from build123d import *

# Parameters (mm, degrees)
SKETCH1_R           = 4.8
SKETCH1_R_2         = 1.5
SKETCH1_R_3         = 4.5
BOSS_EXTRUDE1_DEPTH = 4


with BuildPart() as part:
    # Sketch1 → Boss-Extrude1 (new body)
    # profile 1 of 5: a face of its own
    with BuildSketch(Plane.XY):
        Polygon((-125, 88.228571429), (-125, 63.142246191), (94.856226429, -83.428571429), (123.942857143, -83.428571429), (123.942857143, 88.228571429), align=None)
        with Locations((107.142857143, -71.428571429)):
            Circle(SKETCH1_R, mode=Mode.SUBTRACT)
        with Locations((-107.142857143, 71.428571429)):
            Circle(SKETCH1_R, mode=Mode.SUBTRACT)
        with Locations((21.832408692, 6.152026506)):
            Circle(SKETCH1_R_2, mode=Mode.SUBTRACT)
        with Locations((37.332408692, 21.652026506)):
            Circle(SKETCH1_R_3, mode=Mode.SUBTRACT)
        with Locations((52.832408692, 6.152026506)):
            Circle(SKETCH1_R_2, mode=Mode.SUBTRACT)
        with Locations((21.832408692, 37.152026506)):
            Circle(SKETCH1_R_2, mode=Mode.SUBTRACT)
        with Locations((52.832408692, 37.152026506)):
            Circle(SKETCH1_R_2, mode=Mode.SUBTRACT)
        with Locations((107.142857143, 71.428571429)):
            Circle(SKETCH1_R, mode=Mode.SUBTRACT)
    # profile 2 of 5: a face of its own
    with BuildSketch(Plane.XY):
        with Locations((21.832408692, 6.152026506)):
            Circle(SKETCH1_R_2)
    # profile 3 of 5: a face of its own
    with BuildSketch(Plane.XY):
        with Locations((21.832408692, 37.152026506)):
            Circle(SKETCH1_R_2)
    # profile 4 of 5: a face of its own
    with BuildSketch(Plane.XY):
        with Locations((52.832408692, 37.152026506)):
            Circle(SKETCH1_R_2)
    # profile 5 of 5: a face of its own
    with BuildSketch(Plane.XY):
        with Locations((52.832408692, 6.152026506)):
            Circle(SKETCH1_R_2)
    extrude(amount=BOSS_EXTRUDE1_DEPTH)


solid = part.part
Could you check a few things on this model? Use its own coordinates, in mm. Give positions to 0.01 mm unless a question says otherwise; leave off trailing zeros. Order: outer loops, then holes, each group sorted by start corner. A loop starts at its lowest first (then second) coordinate and runs counter-clockwise, first axis right, second up.
Item 1: I need wall thicknesses on line 1 (Y direction, x = 110.5, z = 0.9); line 2 (X direction, y = 48, z = 3.25); line 3 (X direction, y = 63, z = 3.85). Which ranges of each line are inside material? Lowest first, please.
Item 2: If we section it at A-A, the plane z = 1.6: Write out the boundary of the cut face in (x, y), plus the area to 3 significant figures.
Item 3: If we section it at B-B, the plane y = 31: Write out the boundary of the cut face in (x, z).
Item 4: I'm going to push a flat-ended pin straight in: pin 1 (1 mm diameter, centred on x = 81.5, z = 3.5, fed in from -Y). Where does the tip first touch, or does it pass through?
Item 5: If we section it at C-C, the plane x = -79: Write out the boundary of the cut face in (y, z), plus the area to 3 significant figures.
Item 6: If we mould it in two halves opening along Y, with no side actions, what happens to faces 1 (the face through (-16.61, -9.12, 1.97)), 2 (the face through (36.36, 17.26, 1.97)), 3 (the face through (25, 23, 0))? For each: pulls with the +Y half, pulls with the -Y half, needs draft (parallel to the pull), parting line crosses it, or undercut.
Values:
1. line 1: y = -83.43 to -74.86, -68 to 68, 74.86 to 88.23
1. line 2: x = -102.29 to 123.94
1. line 3: x = -124.79 to 123.94
2. outline: (-125, 63.14) - (94.86, -83.43) - (123.94, -83.43) - (123.94, 88.23) - (-125, 88.23) - close; hole circle Ø9.6 at (-107.14, 71.43); hole circle Ø9 at (37.33, 21.65); hole circle Ø9.6 at (107.14, -71.43); hole circle Ø9.6 at (107.14, 71.43)
2. area: 26,300 mm2
3. outline: (-76.79, 0) - (123.94, 0) - (123.94, 4) - (-76.79, 4) - close
4. pin 1: stops at y = -74.86
5. outline: (32.48, 0) - (88.23, 0) - (88.23, 4) - (32.48, 4) - close
5. area: 223 mm2
6. face 1: pulls with the -Y half
6. face 2: undercut
6. face 3: needs draft
